For this review, take the finished solid that the model builds, in its own axes (mm). A direction names the side the tool comes from. Round coordinates to 2 decimals unless told otherwise and drop trailing zeros. Loops run counter-clockwise (first coordinate to the right, second up) from the corner with the lowest first, then second, coordinate; pieces in that order, holes last. Notation, with made-up numbers: M 4.5,2 L 35.5,2 A15 ccw 35.5,12 Z; hole C 40.5,-38 d5. An arc over 180 degrees is marked long. One line per question, with ' | ' between items. Start each with the question number.
1) For pin 1 Ø3.5 at (y, z) = (43.5, 12.5) entering from +X; pin 2 Ø6 at (y, z) = (43.5, -12.5) entering from +X; pin 3 Ø1.5 at (x, z) = (-6, 0.5) entering from +Y, all flat-tipped, find the tip position at first contact; note any pin that passes through.
2) We need section A-A (x = 0). Give the boundary of the cut face in (y, z), and give its area (3 significant figures).
3) We need section D-D (y = 18.5). Give the boundary of the cut face in (x, z), and give its area (3 significant figures).
4) We need section C-C (x = 17.5). Give the boundary of the cut face in (y, z), and give its area (3 significant figures).
5) For faces 5 (the face through (5.21, 45.73, 12.79)), 6 (the face through (-7.81, 30.57, -1.73)), list the 3-axis set-ups (+Z, -Z, +X, -X, +Y, -Y) from which the entire face can be reached by the end or side of a thin tool; tool diameter is ignored.
6) For probe 1 along Y at (x, z) = (8.25, 12.5); probe 2 along Z at (x, y) = (4, 43); probe 3 along Y at (x, z) = (5, 11), list the stretches that pass through material, from the lowest coordinate up. Write a range as from..to.
7) Mouldability with a two-part tool opening along Y and no side actions: class faces 1 (the face through (-20, 31, 0)), 2 (the face through (9, 0, 0)), 3 (the face through (9, 62, 0)), 4 (the face through (-10, 19, 13)) as pulls with the +Y half, pulls with the -Y half, needs draft (parallel to the pull), parting line crosses it, or undercut.
8) We need section B-B (z = 0). Give the boundary of the cut face in (x, y).
```python
from build123d import *

# Parameters (mm, degrees)
CROQUIS1_W              = 40
CROQUIS1_H              = 48
CROQUIS1_R              = 8
SALIENTE_EXTRUIR1_DEPTH = 62
CROQUIS2_R              = 2.25
CORTAR_EXTRUIR1_DEPTH   = 30


with BuildPart() as part:
    # Croquis1 → Saliente-Extruir1 (new body)
    with BuildSketch(Plane(origin=(0, 0, 0), x_dir=(1, 0, 0), z_dir=(0, 1, 0))):
        Rectangle(CROQUIS1_W, CROQUIS1_H)
        with Locations(Location((0, 0, 0), (0, 0, 270))):
            Circle(CROQUIS1_R, mode=Mode.SUBTRACT)
    extrude(amount=SALIENTE_EXTRUIR1_DEPTH)

    # Croquis2 → Cortar-Extruir1 (cut)
    with BuildSketch(Plane(origin=(20, 0, 0), x_dir=(0, 0, -1), z_dir=(1, 0, 0))):
        with Locations((-12.5, 43.5)):
            Circle(CROQUIS2_R)
        with Locations((12.5, 43.5)):
            Circle(CROQUIS2_R)
        with Locations((-12.5, 18.5)):
            Circle(CROQUIS2_R)
        with Locations((12.5, 18.5)):
            Circle(CROQUIS2_R)
    extrude(amount=-CORTAR_EXTRUIR1_DEPTH, mode=Mode.SUBTRACT)


solid = part.part
```
Answers below:
1) pin 1: x = -10 | pin 2: x = 20 | pin 3: through
2) outline: M 0,-24 L 62,-24 L 62,-8 L 0,-8 Z; M 0,8 L 62,8 L 62,24 L 0,24 Z; hole C 18.5,-12.5 d4.5; hole C 18.5,12.5 d4.5; hole C 43.5,-12.5 d4.5; hole C 43.5,12.5 d4.5 | area: 1,920 mm^2
3) outline: M -20,-24 L 20,-24 L 20,-14.75 L -10,-14.75 L -10,-10.25 L 20,-10.25 L 20,10.25 L -10,10.25 L -10,14.75 L 20,14.75 L 20,24 L -20,24 Z; hole C 0,0 d16 | area: 1,450 mm^2
4) outline: M 0,-24 L 62,-24 L 62,24 L 0,24 Z; hole C 18.5,-12.5 d4.5; hole C 18.5,12.5 d4.5; hole C 43.5,-12.5 d4.5; hole C 43.5,12.5 d4.5 | area: 2,910 mm^2
5) face 5: +X | face 6: +Y, -Y
6) probe 1: 0..16.25, 20.75..41.25, 45.75..62 | probe 2: -24..-14.69, -10.31..-6.93, 6.93..10.31, 14.69..24 | probe 3: 0..16.82, 20.18..41.82, 45.18..62
7) face 1: needs draft | face 2: pulls with the -Y half | face 3: pulls with the +Y half | face 4: undercut
8) outline: M -20,0 L -8,0 L -8,62 L -20,62 Z; M 8,0 L 20,0 L 20,62 L 8,62 Z
